```python
from build123d import *

# Parameters (mm, degrees)
BOSS_EXTRUDE1_DEPTH = 2


with BuildPart() as part:
    # Sketch1 → Boss-Extrude1 (new body)
    with BuildSketch(Plane.XY):
        with BuildLine():
            Line((4, 6), (12.2, 6))
            Line((12.2, 6), (12.2, 5))
            ThreePointArc((12.2, 5), (13.2, 3), (14.2, 5))
            Line((14.2, 5), (14.2, 6))
            Line((14.2, 6), (15.2, 6))
            ThreePointArc((15.2, 6), (15.907106781, 5.707106781), (16.2, 5))
            Line((16.2, 5), (16.2, 0))
            Line((16.2, 0), (12.2, 0))
            Line((12.2, 0), (12.2, 2))
            Line((12.2, 2), (4, 2))
            Line((4, 2), (4, 0))
            Line((4, 0), (0, 0))
            Line((0, 0), (0, 5))
            ThreePointArc((0, 5), (0.292893219, 5.707106781), (1, 6))
            Line((1, 6), (2, 6))
            Line((2, 6), (2, 5))
            ThreePointArc((2, 5), (3, 3), (4, 5))
            Line((4, 5), (4, 6))
        make_face()
    extrude(amount=BOSS_EXTRUDE1_DEPTH)


solid = part.part
```
Verification items for the finished model (mm, model axes). A direction names the side the tool comes from. Coordinates: 2 decimals unless noted, no trailing zeros. Loops run counter-clockwise (first coordinate to the right, second up) from the corner with the lowest first, then second, coordinate; pieces in that order, holes last. Notation, with made-up numbers: (-19, 14) -> (10, 14) arc R24 cw to (10, 26) -> close; hole circle Ø7 at (56, 60.5). An arc over 180 degrees is marked (long way). Answer in a Markdown table with one row per item.
1) Section check D-D (x = 3). Record the cut outline in (y, z), and give its area (3 significant figures).
The answers:
| item | result |
|---|---|
| outline | (0, 0) -> (3, 0) -> (3, 2) -> (0, 2) -> close |
| area | 6.00 mm2 |
2) Access from +Z, -Z, +X, -X, +Y, -Y to the whole of each face (thin tool, end or side, straight path). Record for faces 1 (the face through (15.899, 5.715, 0.986)), 2 (the face through (4, 1, 1)), 3 (the face through (4, 5.5, 1)).
The answers:
| item | result |
|---|---|
| face 1 | +Z, -Z, +X, +Y |
| face 2 | +Z, -Z, -Y |
| face 3 | +Z, -Z, +Y |
3) Section check B-B (y = 4.25). Record the cut outline in (x, z), and give its area (3 significant figures).
The answers:
| item | result |
|---|---|
| outline | (0, 0) -> (1.75, 0) -> (1.75, 2) -> (0, 2) -> close; (4.25, 0) -> (11.95, 0) -> (11.95, 2) -> (4.25, 2) -> close; (14.45, 0) -> (16.2, 0) -> (16.2, 2) -> (14.45, 2) -> close |
| area | 22.4 mm2 |
4) Draft check along X on faces 4 (the face through (1.5, 6, 1)), 5 (the face through (0, 2, 1)), 6 (the face through (12.2, 1, 1)). Enter one of: released by +X, released by -X, zero draft, split by the parting line, or undercut.
The answers:
| item | result |
|---|---|
| face 4 | zero draft |
| face 5 | released by -X |
| face 6 | undercut |
5) Depth check by flat-ended pin: P1, Ø2, axis at x = 3, y = 4.25, coming from the +Z side; P2, Ø0.8, axis at y = 5.5, z = 1.5, coming from the +X side (3 decimals). Enter the tip coordinate at first touch or a pass-through.
The answers:
| item | result |
|---|---|
| P1 | passes through |
| P2 | stops at x = 16.195 |
6) Section check A-A (y = 1.75). Record the cut outline in (x, z).
The answers:
| item | result |
|---|---|
| outline | (0, 0) -> (4, 0) -> (4, 2) -> (0, 2) -> close; (12.2, 0) -> (16.2, 0) -> (16.2, 2) -> (12.2, 2) -> close |
7) Scan lines: line 1 along X through (y, z) = (4.25, 0.4); line 2 along X through (y, z) = (1.3, 0.65); line 3 along X through (y, z) = (3.3, 0.55). Record each from-to range of solid material in increasing order. Write a range as from..to.
The answers:
| item | result |
|---|---|
| line 1 | x = 0..1.75, 4.25..11.95, 14.45..16.2 |
| line 2 | x = 0..4, 12.2..16.2 |
| line 3 | x = 0..2.19, 3.81..12.39, 14.01..16.2 |
8) Section check C-C (z = 0.3). Record the cut outline in (x, y).
The answers:
| item | result |
|---|---|
| outline | (0, 0) -> (4, 0) -> (4, 2) -> (12.2, 2) -> (12.2, 0) -> (16.2, 0) -> (16.2, 5) arc R1 ccw to (15.2, 6) -> (14.2, 6) -> (14.2, 5) arc R1.25 cw (long way) to (12.2, 5) -> (12.2, 6) -> (4, 6) -> (4, 5) arc R1.25 cw (long way) to (2, 5) -> (2, 6) -> (1, 6) arc R1 ccw to (0, 5) -> close |
